Build history of the part. All positions in model axes, mm. A direction names the side the tool comes from. Round coordinates to 2 decimals unless told otherwise and drop trailing zeros. Loops run counter-clockwise (first coordinate to the right, second up) from the corner with the lowest first, then second, coordinate; pieces in that order, holes last. Notation, with made-up numbers: M 73.5,48.5 L 123.5,48.5 A5 cw 123.5,56.5 Z; hole C 88,54.5 d3. An arc over 180 degrees is marked long. One line per item, written item: value.
```python
from build123d import *

# Parameters (mm, degrees)
SKETCH4_W           = 47
SKETCH4_H           = 40
SKETCH4_R           = 1.27
BOSS_EXTRUDE1_DEPTH = 1
FILLET1_R           = 7
SKETCH5_W           = 11.6
SKETCH5_H           = 15
BOSS_EXTRUDE2_DEPTH = 2.5
SKETCH6_W           = 5.6
SKETCH6_H           = 10.9
BOSS_EXTRUDE3_DEPTH = 4.5
SKETCH7_W           = 25
SKETCH7_H           = 25
BOSS_EXTRUDE4_DEPTH = 4
FILLET2_R           = 4
SKETCH8_R           = 1.75
BOSS_EXTRUDE5_DEPTH = 0.2
FILLET3_R           = 0.5
SKETCH9_W           = 8
SKETCH9_H           = 5.5
BOSS_EXTRUDE6_DEPTH = 2.4
FILLET4_R           = 0.5


with BuildPart() as part:
    # Sketch4 → Boss-Extrude1 (new body)
    with BuildSketch(Plane(origin=(0, 0, 0), x_dir=(1, 0, 0), z_dir=(0, 1, 0))):
        Rectangle(SKETCH4_W, SKETCH4_H)
        with Locations(Location((16.23, -16.13, 0), (0, 0, 270))):
            Circle(SKETCH4_R, mode=Mode.SUBTRACT)
        with Locations(Location((-17.23, -16.13, 0), (0, 0, 270))):
            Circle(SKETCH4_R, mode=Mode.SUBTRACT)
        with Locations(Location((-17.23, 15.93, 0), (0, 0, 270))):
            Circle(SKETCH4_R, mode=Mode.SUBTRACT)
        with BuildLine():
            Line((13.77, 14.66), (16.23, 14.66))
            ThreePointArc((16.23, 14.66), (17.5, 15.93), (16.23, 17.2))
            Line((16.23, 17.2), (13.77, 17.2))
            ThreePointArc((13.77, 17.2), (12.5, 15.93), (13.77, 14.66))
        make_face(mode=Mode.SUBTRACT)
    extrude(amount=BOSS_EXTRUDE1_DEPTH)

    # Fillet1
    fillet1_edges = [part.edges().sort_by_distance(p)[0] for p in [
        (23.5, 0.5, -20),
        (23.5, 0.5, 20),
        (-23.5, 0.5, 20),
        (-23.5, 0.5, -20),
    ]]
    fillet(fillet1_edges, radius=FILLET1_R)

    # Sketch5 → Boss-Extrude2 (add)
    with BuildSketch(Plane.XZ):
        with Locations((11, 3.6)):
            Rectangle(SKETCH5_W, SKETCH5_H)
    extrude(amount=BOSS_EXTRUDE2_DEPTH)

    # Sketch6 → Boss-Extrude3 (add)
    with BuildSketch(Plane.XZ):
        with Locations((-17.7, -4.55)):
            Rectangle(SKETCH6_W, SKETCH6_H)
    extrude(amount=BOSS_EXTRUDE3_DEPTH)

    # Sketch7 → Boss-Extrude4 (add)
    with BuildSketch(Plane(origin=(0, 1, 0), x_dir=(1, 0, 0), z_dir=(0, 1, 0))):
        with Locations((-0.6, -2.6)):
            Rectangle(SKETCH7_W, SKETCH7_H)
    extrude(amount=BOSS_EXTRUDE4_DEPTH)

    # Fillet2
    fillet2_edges = [part.edges().sort_by_distance(p)[0] for p in [
        (-13.1, 3, -9.9),
        (-13.1, 3, 15.1),
        (11.9, 3, 15.1),
        (11.9, 3, -9.9),
    ]]
    fillet(fillet2_edges, radius=FILLET2_R)

    # Sketch8 → Boss-Extrude5 (add)
    with BuildSketch(Plane(origin=(0, 5, 0), x_dir=(1, 0, 0), z_dir=(0, 1, 0))):
        with Locations(Location((-0.6, -0.4, 0), (0, 0, 270))):
            Circle(SKETCH8_R)
    extrude(amount=BOSS_EXTRUDE5_DEPTH)

    # Fillet3
    # the kernel refuses this fillet: 0.5 mm, written as the material it takes off along each edge
    with BuildSketch(Plane(origin=(-0.6, 5.2, 0.4), x_dir=(0, 0, 1), z_dir=(-1, 0, 0))) as fillet3_piece_1:
        with BuildLine():
            CenterArc((1.35, -0.5), FILLET3_R, 36.869897645, 53.130102355)
            Line((1.35, 0), (1.35, 0.01))
            Line((1.35, 0.01), (1.75, 0.01))
            Line((1.75, 0.01), (1.76, 0))
            ThreePointArc((1.76, 0), (1.76, -0.1), (1.758, -0.194))
            Line((1.758, -0.194), (1.75, -0.2))
        make_face()
    revolve(axis=Axis((-0.6, 5.2, 0.4), (0, 1, 0)), mode=Mode.SUBTRACT)

    # Sketch9 → Boss-Extrude6 (add)
    with BuildSketch(Plane.XZ):
        with Locations((-1, -17.95)):
            Rectangle(SKETCH9_W, SKETCH9_H)
    extrude(amount=BOSS_EXTRUDE6_DEPTH)

    # Fillet4
    fillet4_edges = [part.edges().sort_by_distance(p)[0] for p in [
        (-13.1, 5, 2.6),
        (-0.6, 5, -9.9),
        (-0.6, 5, 15.1),
        (11.9, 5, 2.6),
        (10.728427125, 5, -8.728427125),
        (10.728427125, 5, 13.928427125),
        (-11.928427125, 5, 13.928427125),
        (-11.928427125, 5, -8.728427125),
    ]]
    fillet(fillet4_edges, radius=FILLET4_R)


solid = part.part
```
Item 1: Wall check: line 1 along X through (y, z) = (0.6, 16.13); line 2 along Y through (x, z) = (15.5, -1); line 3 along Y through (x, z) = (-15.5, -16). Give the ranges that are in metal, low to high.
Check values:
line 1: x = -22.76 to -18.5, -15.96 to 14.96, 17.5 to 22.76
line 2: y = -2.5 to 1
line 3: y = 0 to 1
Item 2: Slice it at D-D, the plane y = 2.75. Give the cut face in (x, z).
Check values:
outline: M -13.1,-5.9 A4 ccw -9.1,-9.9 L 7.9,-9.9 A4 ccw 11.9,-5.9 L 11.9,11.1 A4 ccw 7.9,15.1 L -9.1,15.1 A4 ccw -13.1,11.1 Z
Item 3: Slice it at B-B, the plane z = -15.93. Give the cut face in (x, y), and give its area (3 significant figures).
Check values:
outline: M -22.86,0 L -18.5,0 L -18.5,1 L -22.86,1 Z; M -15.96,0 L -5,0 L -5,-2.4 L 3,-2.4 L 3,0 L 12.5,0 L 12.5,1 L -15.96,1 Z; M 17.5,0 L 22.86,0 L 22.86,1 L 17.5,1 Z
area: 57.4 mm2
Item 4: Slice it at C-C, the plane x = -17.23. Give the cut face in (y, z), and give its area (3 significant figures).
Check values:
outline: M -4.5,-10 L 0,-10 L 0,-14.66 L 1,-14.66 L 1,14.86 L 0,14.86 L 0,0.9 L -4.5,0.9 Z; M 0,-19.96 L 1,-19.96 L 1,-17.2 L 0,-17.2 Z; M 0,17.4 L 1,17.4 L 1,19.96 L 0,19.96 Z
area: 83.9 mm2
Item 5: Drop flat-ended pins along their axis: P1, Ø1.9, axis at y = -1.5, z = -17.5, coming from the +X side; P2, Ø12, axis at x = -4.5, z = -2, coming from the -Y side; P3, Ø3, axis at y = 2, z = 4.5, coming from the -X side; P4, Ø1.5, axis at x = 11, y = -2.5, coming from the -Z side. Give the stop position or say it passes through.
Check values:
P1: stops at x = 3
P2: stops at y = 0
P3: stops at x = -23.5
P4: stops at z = -3.9
Item 6: Pull direction Z, two halves, no side cores. Call faces 4 (the face through (-1, 3, -9.9)), 5 (the face through (-1, -1, -15.2)), 6 (the face through (17.088, 0.493, 15.194)): pulls with the +Z half, pulls with the -Z half, needs draft (parallel to the pull), parting line crosses it, or undercut.
Check values:
face 4: pulls with the -Z half
face 5: pulls with the +Z half
face 6: undercut
Item 7: Which spindle directions (+Z, -Z, +X, -X, +Y, -Y) get a long thin tool onto all of the face, cutting with end or side? Do faces 1 (the face through (-11.897, 2.774, 13.959)), 2 (the face through (-20.5, -2, -5)), 3 (the face through (17.5, 0.5, -15.9)). Say none if no direction does.
Check values:
face 1: +Z, -X, +Y
face 2: +Z, -Z, -X, -Y
face 3: +Y, -Y
Item 8: Slice it at A-A, the plane y = -1.5. Give the cut face in (x, z).
Check values:
outline: M -20.5,-10 L -14.9,-10 L -14.9,0.9 L -20.5,0.9 Z; M -5,-20.7 L 3,-20.7 L 3,-15.2 L -5,-15.2 Z; M 5.2,-3.9 L 16.8,-3.9 L 16.8,11.1 L 5.2,11.1 Z
